For this review, take the finished solid that the model builds, in its own axes (mm). Face numbers are marked on the shaded views. A direction names the side the tool comes from. Coordinates: 2 decimals unless noted, no trailing zeros. Write each loop counter-clockwise with the first axis right and the second up, starting at its lowest first coordinate (ties: lowest second). Pieces come first, ordered by that corner, then holes. Notation, with made-up numbers: (74, -13) -> (83, -13) arc R27 ccw to (83, 19) -> close; hole circle Ø7 at (-13, -17.75). An arc over 180 degrees is marked (long way). One line per item, written item: value. Start each with the question number.
1) Machinability: for the marked faces 1 and 2, which of the approach directions +Z, -Z, +X, -X, +Y, -Y give a long, thin tool a straight path to every point of the face, cutting with its end or side? Answer none if there is none.
2) Add section A-A (x = -2.25). State the section outline as (y, z) points.
3) Add section C-C (z = 2.75). State how many separate pieces and enclosed holes the cut face has, and give its area (3 significant figures).
4) Add section B-B (y = -4). State the section outline as (x, z) points, and give its area (3 significant figures).
5) Mouldability with a two-part tool opening along X and no side actions: class the marked faces 3, 4 and 5 as released by +X, released by -X, zero draft, split by the parting line, or undercut.
6) For pin 1 Ø1.5 at (x, y) = (-0.5, -4.5) entering from +Z, flat-tipped, find the tip position at first contact; note if it passes through.
7) For probe 1 along X at (y, z) = (-0.5, -0.75) (1 decimal); probe 2 along X at (y, z) = (-1.5, 2); probe 3 along Z at (x, y) = (-1.5, -3.75), list the stretches that pass through material, from the lowest coordinate up. Write a range as from..to.
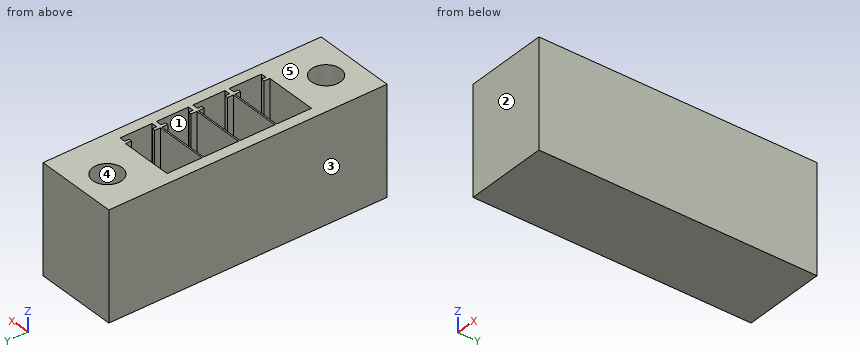
from build123d import *

# Parameters (mm, degrees)
SKETCH1_W           = 9.398
SKETCH1_H           = 24.2316
BOSS_EXTRUDE1_DEPTH = 7.239
HOLE1_D             = 2.54
HOLE1_DEPTH         = 6.35
HOLE1_TIP           = 0.763092986
CUT_EXTRUDE1_REACH  = 16.15


with BuildPart() as part:
    # Sketch1 → Boss-Extrude1 (new body)
    with BuildSketch(Plane(origin=(3.6195, 0, 0), x_dir=(0, 0, -1), z_dir=(1, 0, 0))):
        Rectangle(SKETCH1_W, SKETCH1_H)
    extrude(amount=-BOSS_EXTRUDE1_DEPTH)

    # Hole1
    with Locations(Plane.XY.offset(4.699)):
        with Locations((-0.1905, -9.525), (-0.1905, 9.525)):
            Hole(HOLE1_D / 2, depth=HOLE1_DEPTH)
            with Locations((0, 0, -(HOLE1_DEPTH + HOLE1_TIP / 2))):  # 118° drill point
                Cone(0, HOLE1_D / 2, HOLE1_TIP, mode=Mode.SUBTRACT)

    # Sketch4 → Cut-Extrude1 (cut, up to next)
    with BuildSketch(Plane(origin=(0, 0, -1.651), x_dir=(-1, 0, 0), z_dir=(0, 0, -1)), mode=Mode.PRIVATE) as cut_extrude1_sk1:
        Polygon((2.667, 6.2865), (-1.905, 6.2865), (-1.905, 5.7785), (-2.159, 5.7785), (-2.159, 6.1595), (-2.667, 6.1595), (-2.667, 3.3655), (-2.159, 3.3655), (-2.159, 3.7465), (-1.905, 3.7465), (-1.905, 3.2385), (2.667, 3.2385), align=None)
    cut_extrude1_tool1 = extrude(cut_extrude1_sk1.sketch, amount=-CUT_EXTRUDE1_REACH, mode=Mode.PRIVATE) & part.part
    # Sketch4 → Cut-Extrude1 (cut, up to next)
    with BuildSketch(Plane(origin=(0, 0, -1.651), x_dir=(-1, 0, 0), z_dir=(0, 0, -1)), mode=Mode.PRIVATE) as cut_extrude1_sk2:
        Polygon((2.667, 3.1115), (-1.905, 3.1115), (-1.905, 2.6035), (-2.159, 2.6035), (-2.159, 2.9845), (-2.667, 2.9845), (-2.667, 0.1905), (-2.159, 0.1905), (-2.159, 0.5715), (-1.905, 0.5715), (-1.905, 0.0635), (2.667, 0.0635), align=None)
    cut_extrude1_tool2 = extrude(cut_extrude1_sk2.sketch, amount=-CUT_EXTRUDE1_REACH, mode=Mode.PRIVATE) & part.part
    # Sketch4 → Cut-Extrude1 (cut, up to next)
    with BuildSketch(Plane(origin=(0, 0, -1.651), x_dir=(-1, 0, 0), z_dir=(0, 0, -1)), mode=Mode.PRIVATE) as cut_extrude1_sk3:
        Polygon((2.667, -0.0635), (-1.905, -0.0635), (-1.905, -0.5715), (-2.159, -0.5715), (-2.159, -0.1905), (-2.667, -0.1905), (-2.667, -2.9845), (-2.159, -2.9845), (-2.159, -2.6035), (-1.905, -2.6035), (-1.905, -3.1115), (2.667, -3.1115), align=None)
    cut_extrude1_tool3 = extrude(cut_extrude1_sk3.sketch, amount=-CUT_EXTRUDE1_REACH, mode=Mode.PRIVATE) & part.part
    # Sketch4 → Cut-Extrude1 (cut, up to next)
    with BuildSketch(Plane(origin=(0, 0, -1.651), x_dir=(-1, 0, 0), z_dir=(0, 0, -1)), mode=Mode.PRIVATE) as cut_extrude1_sk4:
        Polygon((2.667, -3.2385), (-1.905, -3.2385), (-1.905, -3.7465), (-2.159, -3.7465), (-2.159, -3.3655), (-2.667, -3.3655), (-2.667, -6.1595), (-2.159, -6.1595), (-2.159, -5.7785), (-1.905, -5.7785), (-1.905, -6.2865), (2.667, -6.2865), align=None)
    cut_extrude1_tool4 = extrude(cut_extrude1_sk4.sketch, amount=-CUT_EXTRUDE1_REACH, mode=Mode.PRIVATE) & part.part
    add(cut_extrude1_tool1.solids().sort_by_distance((-0.052659, 4.7625, -1.651))[0], mode=Mode.SUBTRACT)
    add(cut_extrude1_tool2.solids().sort_by_distance((-0.052659, 1.5875, -1.651))[0], mode=Mode.SUBTRACT)
    add(cut_extrude1_tool3.solids().sort_by_distance((-0.052659, -1.5875, -1.651))[0], mode=Mode.SUBTRACT)
    add(cut_extrude1_tool4.solids().sort_by_distance((-0.052659, -4.7625, -1.651))[0], mode=Mode.SUBTRACT)


solid = part.part
Numbers:
1. face 1: +Z
1. face 2: +Z, -Z, +X, -X, -Y
2. outline: (-12.12, -4.7) -> (12.12, -4.7) -> (12.12, 4.7) -> (6.29, 4.7) -> (6.29, -1.65) -> (3.24, -1.65) -> (3.24, 4.7) -> (3.11, 4.7) -> (3.11, -1.65) -> (0.06, -1.65) -> (0.06, 4.7) -> (-0.06, 4.7) -> (-0.06, -1.65) -> (-3.11, -1.65) -> (-3.11, 4.7) -> (-3.24, 4.7) -> (-3.24, -1.65) -> (-6.29, -1.65) -> (-6.29, 4.7) -> (-12.12, 4.7) -> close
3. separate pieces: 1
3. enclosed holes: 6
3. area: 102 mm²
4. outline: (-3.62, -4.7) -> (3.62, -4.7) -> (3.62, 4.7) -> (2.67, 4.7) -> (2.67, -1.65) -> (-2.67, -1.65) -> (-2.67, 4.7) -> (-3.62, 4.7) -> close
4. area: 34.2 mm²
5. face 3: released by -X
5. face 4: undercut
5. face 5: zero draft
6. pin 1: z = -1.65
7. probe 1: -3.6..-2.7, 1.9..2.2, 2.7..3.6
7. probe 2: -3.62..-2.67, 2.67..3.62
7. probe 3: -4.7..-1.65
